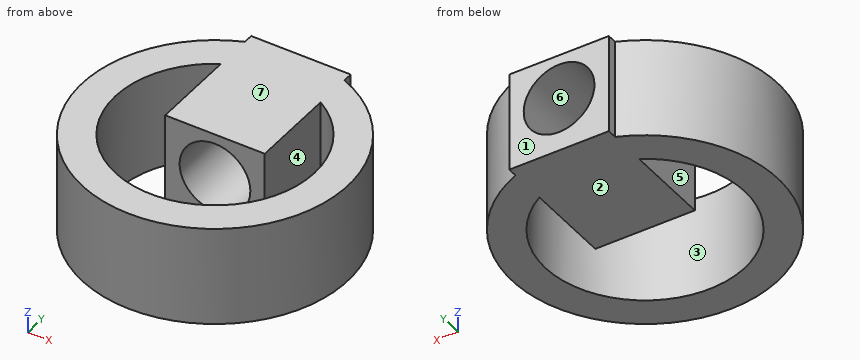
from build123d import *

# Parameters (mm, degrees)
SKETCH2_R               = 25.4
BOSS_EXTRUDE1_DEPTH     = 19.05
CUT_EXTRUDE1_DEPTH      = 41.659838908
CUT_EXTRUDE1_DEPTH_BACK = 41.659838908
SKETCH3_R               = 19.05
SKETCH4_W               = 19.05
SKETCH4_H               = 19.05
BOSS_EXTRUDE2_DEPTH     = 25.4
SKETCH7_R               = 6.769739398
CUT_EXTRUDE2_DEPTH      = 41.659838908


with BuildPart() as part:
    # Sketch2 → Boss-Extrude1 (new body)
    with BuildSketch(Plane.XY):
        with Locations(Location((0, 0, 0), (0, 0, 180))):
            Circle(SKETCH2_R)
    extrude(amount=BOSS_EXTRUDE1_DEPTH)

    # Sketch3 → Cut-Extrude1 (cut, two sides: drawn at the far end of the back side and taken through both)
    with BuildSketch(Plane.XY.offset(19.05).offset(-CUT_EXTRUDE1_DEPTH_BACK)):
        Circle(SKETCH3_R)
    extrude(amount=CUT_EXTRUDE1_DEPTH + CUT_EXTRUDE1_DEPTH_BACK, mode=Mode.SUBTRACT)

    # Sketch4 → Boss-Extrude2 (add)
    with BuildSketch(Plane(origin=(0, 0, 0), x_dir=(1, 0, 0), z_dir=(0, 1, 0))):
        with Locations((0, -9.525)):
            Rectangle(SKETCH4_W, SKETCH4_H)
    extrude(amount=BOSS_EXTRUDE2_DEPTH)

    # Sketch7 → Cut-Extrude2 (cut, through all)
    with BuildSketch(Plane(origin=(0, 0, 0), x_dir=(1, 0, 0), z_dir=(0, 1, 0))):
        with Locations(Location((0, -10.42763192, 0), (0, 0, 270))):
            Circle(SKETCH7_R)
    extrude(amount=CUT_EXTRUDE2_DEPTH, mode=Mode.SUBTRACT)


solid = part.part
Verification items for the finished model (mm, model axes). Face numbers are marked on the shaded views. A direction names the side the tool comes from. Round coordinates to 2 decimals unless told otherwise and drop trailing zeros. Order: outer loops, then holes, each group sorted by start corner. A loop starts at its lowest first (then second) coordinate and runs counter-clockwise, first axis right, second up. Notation, with made-up numbers: (-36.5, -10) -> (-23.5, -10) arc R19 cw to (-23.5, -4) -> close; hole circle Ø11 at (-19, 65). An arc over 180 degrees is marked (long way). Put each result on its own line as item: value.
1) Depth check by flat-ended pin: pin 1 (3 mm diameter, centred on y = 9.5, z = 9, fed in from -X); pin 2 (0.9 mm diameter, centred on y = 25, z = 10, fed in from -X) (3 decimals); pin 3 (1 mm diameter, centred on x = -1.5, z = 6.5, fed in from +Y). Enter the tip coordinate at first touch or a pass-through.
Final values:
pin 1: stops at x = -24.11
pin 2: stops at x = -9.525
pin 3: stops at y = -18.94
2) Material ranges on line 1 (X direction, y = -0.5, z = 17.5); line 2 (X direction, y = 10.5, z = 16.25) (3 decimals); line 3 (Z direction, x = 0, y = 9), recorded low to high.
Final values:
line 1: x = -25.4 to -19.04, 19.04 to 25.4
line 2: x = -23.128 to -15.895, -9.525 to -3.454, 3.454 to 9.525, 15.895 to 23.128
line 3: z = 0 to 3.66, 17.2 to 19.05
3) Mould release check, pull along Y, two halves, no side actions. Record for the marked faces 1, 2, 3 and 4: +Y half, -Y half, draft (parallel to the pull), parting line (faces both ways), or undercut.
Final values:
face 1: +Y half
face 2: draft
face 3: undercut
face 4: undercut
4) Set-up check for the marked faces 5, 6 and 7: record each of +Z, -Z, +X, -X, +Y, -Y from which the full face is reachable in a straight line by a thin tool's end or side.
Final values:
face 5: +Z, -Z
face 6: +Y
face 7: +Z, +X, -X, +Y, -Y
5) Section check D-D (x = -7.5). Record the cut outline in (y, z).
Final values:
outline: (-24.27, 0) -> (-17.51, 0) -> (-17.51, 19.05) -> (-24.27, 19.05) -> close; (0, 0) -> (25.4, 0) -> (25.4, 19.05) -> (0, 19.05) -> close
6) Section check C-C (y = -14.5). Record the cut outline in (x, z), then the cut area to 3 significant figures.
Final values:
outline: (-20.85, 0) -> (-12.36, 0) -> (-12.36, 19.05) -> (-20.85, 19.05) -> close; (12.36, 0) -> (20.85, 0) -> (20.85, 19.05) -> (12.36, 19.05) -> close
area: 324 mm^2
7) Section check B-B (z = 3). Record the cut outline in (x, y) (3 decimals).
Final values:
outline: (-9.525, 23.546) arc R25.4 ccw (long way) to (9.525, 23.546) -> (9.525, 25.4) -> (-9.525, 25.4) -> close; hole (-9.525, 0) -> (-9.525, 16.498) arc R19.05 ccw (long way) to (9.525, 16.498) -> (9.525, 0) -> close
8) Section check A-A (x = 0). Record the cut outline in (y, z), then the cut area to 3 significant figures.
Final values:
outline: (-25.4, 0) -> (-19.05, 0) -> (-19.05, 19.05) -> (-25.4, 19.05) -> close; (0, 0) -> (25.4, 0) -> (25.4, 3.66) -> (0, 3.66) -> close; (0, 17.2) -> (25.4, 17.2) -> (25.4, 19.05) -> (0, 19.05) -> close
area: 261 mm^2
